```python
from build123d import *

# Parameters (mm, degrees)
SKETCH1_W           = 33
SKETCH1_H           = 25
BOSS_EXTRUDE1_DEPTH = 1
CUT_EXTRUDE1_DEPTH  = 42.412558482
SKETCH3_R           = 0.4
SKETCH3_R_2         = 0.442084783
SKETCH3_R_3         = 0.458227678
CUT_EXTRUDE2_DEPTH  = 42.412558482
BOSS_EXTRUDE3_DEPTH = 2


with BuildPart() as part:
    # Sketch1 → Boss-Extrude1 (new body)
    with BuildSketch(Plane(origin=(0, 0, 0), x_dir=(1, 0, 0), z_dir=(0, 1, 0))):
        with Locations((16.5, 12.5)):
            Rectangle(SKETCH1_W, SKETCH1_H)
    extrude(amount=BOSS_EXTRUDE1_DEPTH)

    # Sketch2 → Cut-Extrude1 (cut, through all)
    with BuildSketch(Plane.XZ):
        Polygon((33, 0), (26.482981269, 0), (33, -7.837809095), align=None)
        Polygon((33, -17.162190905), (33, -25), (26.482981269, -25), align=None)
    extrude(amount=-CUT_EXTRUDE1_DEPTH, mode=Mode.SUBTRACT)

    # Sketch3 → Cut-Extrude2 (cut, through all)
    with BuildSketch(Plane(origin=(0, 1, 0), x_dir=(1, 0, 0), z_dir=(0, 1, 0))):
        with Locations(Location((7.143852183, 23.936106005, 0), (0, 0, 270))):
            Circle(SKETCH3_R)
        with Locations(Location((9.143852183, 23.936106005, 0), (0, 0, 270))):
            Circle(SKETCH3_R)
        with Locations(Location((11.143852183, 23.936106005, 0), (0, 0, 270))):
            Circle(SKETCH3_R)
        with Locations(Location((13.143852183, 23.936106005, 0), (0, 0, 270))):
            Circle(SKETCH3_R)
        with Locations(Location((15.143852183, 23.936106005, 0), (0, 0, 270))):
            Circle(SKETCH3_R)
        with Locations(Location((17.143852183, 23.936106005, 0), (0, 0, 270))):
            Circle(SKETCH3_R)
        with Locations(Location((19.143852183, 23.936106005, 0), (0, 0, 270))):
            Circle(SKETCH3_R)
        with Locations(Location((21.143852183, 23.936106005, 0), (0, 0, 270))):
            Circle(SKETCH3_R)
        with Locations(Location((23.143852183, 23.936106005, 0), (0, 0, 270))):
            Circle(SKETCH3_R)
        with Locations(Location((25.143852183, 23.936106005, 0), (0, 0, 270))):
            Circle(SKETCH3_R)
        with Locations(Location((25.143852183, 1.063893995, 0), (0, 0, 90))):
            Circle(SKETCH3_R)
        with Locations(Location((23.143852183, 1.063893995, 0), (0, 0, 90))):
            Circle(SKETCH3_R)
        with Locations(Location((21.143852183, 1.063893995, 0), (0, 0, 90))):
            Circle(SKETCH3_R)
        with Locations(Location((19.143852183, 1.063893995, 0), (0, 0, 90))):
            Circle(SKETCH3_R)
        with Locations(Location((17.143852183, 1.063893995, 0), (0, 0, 90))):
            Circle(SKETCH3_R)
        with Locations(Location((15.143852183, 1.063893995, 0), (0, 0, 90))):
            Circle(SKETCH3_R)
        with Locations(Location((13.143852183, 1.063893995, 0), (0, 0, 90))):
            Circle(SKETCH3_R)
        with Locations(Location((11.143852183, 1.063893995, 0), (0, 0, 90))):
            Circle(SKETCH3_R)
        with Locations(Location((9.143852183, 1.063893995, 0), (0, 0, 90))):
            Circle(SKETCH3_R)
        with Locations(Location((7.143852183, 1.063893995, 0), (0, 0, 90))):
            Circle(SKETCH3_R)
        with Locations(Location((0.784299075, 22.325061426, 0), (0, 0, 270))):
            Circle(SKETCH3_R_2)
        with Locations(Location((24.152709784, 2.722277331, 0), (0, 0, 270))):
            Circle(SKETCH3_R_3)
    extrude(amount=-CUT_EXTRUDE2_DEPTH, mode=Mode.SUBTRACT)

    # Sketch6 → Boss-Extrude3 (add)
    with BuildSketch(Plane.XZ):
        with BuildLine():
            Line((24.507853381, -22.428957603), (0.778175079, -22.428957603))
            ThreePointArc((0.778175079, -22.428957603), (0.424621688, -22.282510994), (0.278175079, -21.928957603))
            Line((0.278175079, -21.928957603), (0.278175079, -2.903294195))
            ThreePointArc((0.278175079, -2.903294195), (0.424621688, -2.549740805), (0.778175079, -2.403294195))
            Line((0.778175079, -2.403294195), (24.507853381, -2.403294195))
            ThreePointArc((24.507853381, -2.403294195), (24.861406772, -2.549740805), (25.007853381, -2.903294195))
            Line((25.007853381, -2.903294195), (25.007853381, -21.928957603))
            ThreePointArc((25.007853381, -21.928957603), (24.861406772, -22.282510994), (24.507853381, -22.428957603))
        make_face()
    extrude(amount=BOSS_EXTRUDE3_DEPTH)


solid = part.part
```
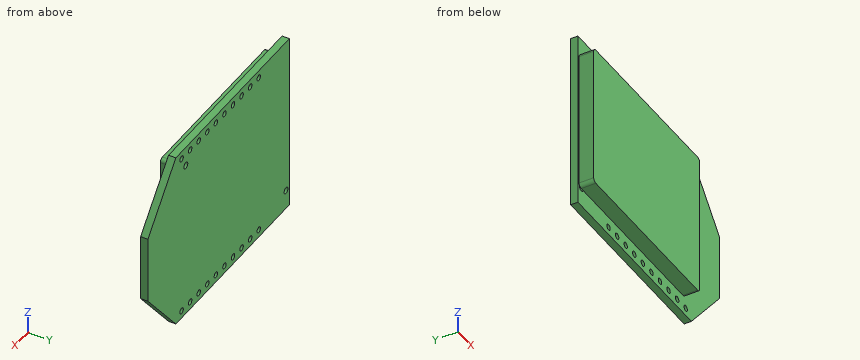
The listing builds one solid part. Answer for the finished solid, in the listing's coordinates (mm). Round coordinates to 2 decimals unless told otherwise and drop trailing zeros. Order: outer loops, then holes, each group sorted by start corner. A loop starts at its lowest first (then second) coordinate and runs counter-clockwise, first axis right, second up. Notation, with made-up numbers: (-40, 33) -> (-9, 33) arc R35 ccw to (-9, 69) -> close; hole circle Ø3 at (-32, -0.5). An arc over 180 degrees is marked (long way). Answer as CSV lines item,"result". Start each with the question number.
(1) The part is cut by section B-B (z = -8.5). Determine the outline of the cut face in (x, y).
(2) The part is cut by section A-A (y = -1.2). Determine the outline of the cut face in (x, z).
(3) Find the intervals of material crossed by probe 1 along Z at (x, y) = (21, -0.8); probe 2 along X at (y, z) = (-1.8, -19); probe 3 along Y at (x, z) = (30, -14), in increasing order. Write a range as from..to.
(4) Flat-ended cylindrical pins translate along their axes: pin 1 Ø1 at (y, z) = (-1.5, -9.5) entering from +X; pin 2 Ø1 at (x, y) = (13.5, -1) entering from +Z; pin 3 Ø1.6 at (y, z) = (-1.5, -9) entering from -X. Find the tip coordinate at first contact, or state that the pin passes through.
(5) The part is cut by section C-C (x = 26). Determine the outline of the cut face in (y, z).
Evaluation:
1,outline,"(0, 0) -> (0.28, 0) -> (0.28, -2) -> (25.01, -2) -> (25.01, 0) -> (33, 0) -> (33, 1) -> (0, 1) -> close"
2,outline,"(0.28, -21.93) arc R0.5 ccw to (0.78, -22.43) -> (24.51, -22.43) arc R0.5 ccw to (25.01, -21.93) -> (25.01, -2.9) arc R0.5 ccw to (24.51, -2.4) -> (0.78, -2.4) arc R0.5 ccw to (0.28, -2.9) -> close"
3,probe 1,"-22.43..-2.4"
3,probe 2,"0.28..25.01"
3,probe 3,"0..1"
4,pin 1,"x = 25.01"
4,pin 2,"z = -2.4"
4,pin 3,"x = 0.28"
5,outline,"(0, -25) -> (1, -25) -> (1, 0) -> (0, 0) -> close"
